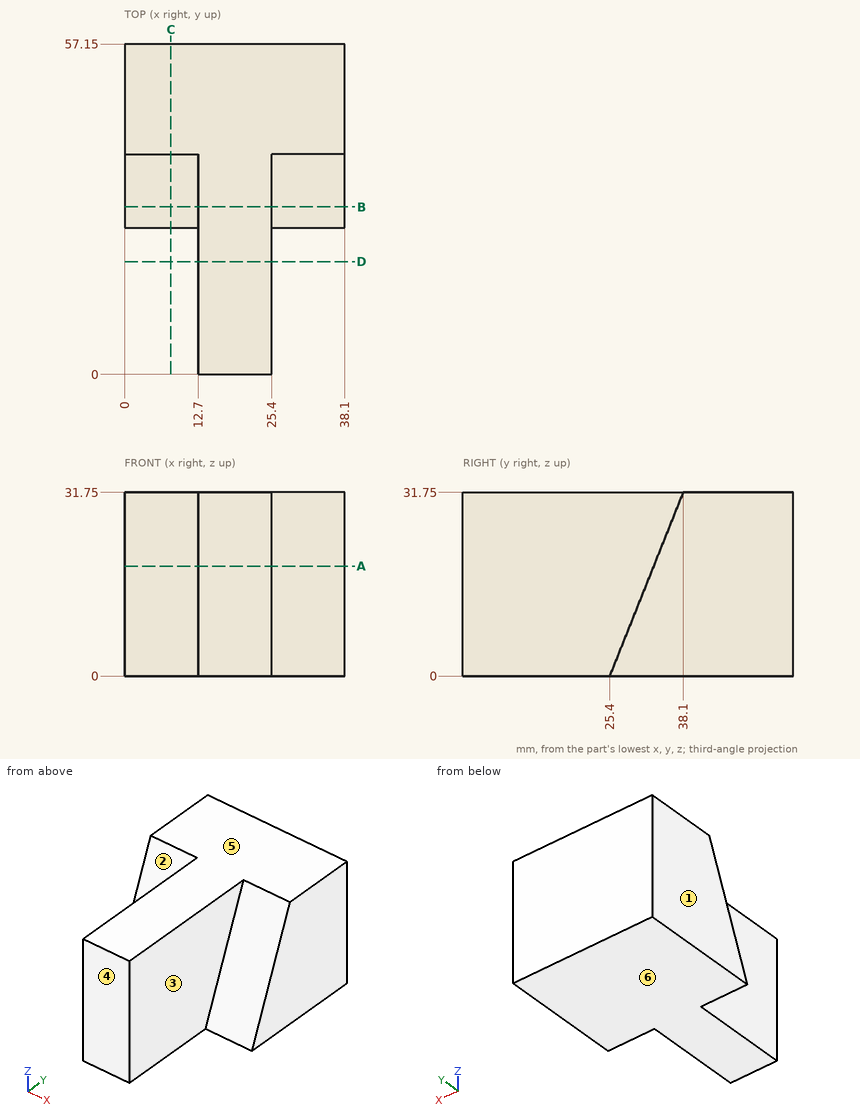
Study the drawing (mm; zero at the part's minimum x, y, z) and answer. A direction names the side the tool comes from. Give positions to 0.01 mm unless a question says otherwise; leave off trailing zeros. Loops run counter-clockwise (first coordinate to the right, second up) from the corner with the lowest first, then second, coordinate; pieces in that order, holes last. Notation, with made-up numbers: M -20,-40 L 36,-40 A26 cw 36,-24 Z; hole C 16.5,-13.75 d8. An arc over 180 degrees is marked long. One line per item, written item: value.
1. Section A-A on z = 19 is taken. Determine the outline of the cut face in (x, y), plus the area to 3 significant figures.
Found:
outline: M 0,33 L 12.7,33 L 12.7,0 L 25.4,0 L 25.4,33 L 38.1,33 L 38.1,57.15 L 0,57.15 Z
area: 1,340 mm^2
2. For a pull along Z with two mould halves and no side action, classify the marked faces 4, 5 and 6 as pulls with the +Z half, pulls with the -Z half, needs draft (parallel to the pull), parting line crosses it, or undercut.
Found:
face 4: needs draft
face 5: pulls with the +Z half
face 6: pulls with the -Z half
3. Section B-B on y = 29 is taken. Determine the outline of the cut face in (x, z).
Found:
outline: M 0,0 L 38.1,0 L 38.1,9 L 25.4,9 L 25.4,31.75 L 12.7,31.75 L 12.7,9 L 0,9 Z
4. Find the intervals of material crossed by probe 1 along X at (y, z) = (26, 4); probe 2 along Y at (x, z) = (7, 13); probe 3 along Y at (x, z) = (9, 20), in increasing order.
Found:
probe 1: 12.7 to 25.4
probe 2: 30.6 to 57.15
probe 3: 33.4 to 57.15
5. This flat-tipped pin is pushed along its axis until it touches: P1, Ø6, axis at y = 24.5, z = 18.5, coming from the -X side. Where does it stop, or does it pass through?
Found:
P1: x = 12.7
6. Section D-D on y = 19.5 is taken. Determine the outline of the cut face in (x, z).
Found:
outline: M 12.7,0 L 25.4,0 L 25.4,31.75 L 12.7,31.75 Z
7. For the marked faces 1, 2 and 3, determine the directions among +Z, -Z, +X, -X, +Y, -Y from which every point of the face is accessible in a straight line to the end or side of a thin tool.
Found:
face 1: +Z, -Z, -X, +Y, -Y
face 2: +Z, -X, -Y
face 3: +Z, +X, -Y
8. Section C-C on x = 8 is taken. Determine the outline of the cut face in (y, z), plus the area to 3 significant figures.
Found:
outline: M 25.4,0 L 57.15,0 L 57.15,31.75 L 38.1,31.75 Z
area: 806 mm^2
